Read the model definition and answer for the solid it produces. Units are mm, in the model's axes. A direction names the side the tool comes from. Coordinates: 2 decimals unless noted, no trailing zeros. Write each loop counter-clockwise with the first axis right and the second up, starting at its lowest first coordinate (ties: lowest second). Pieces come first, ordered by that corner, then holes. Notation, with made-up numbers: (76.5, 86.25) -> (130.5, 86.25) arc R29 ccw to (130.5, 120.25) -> close; hole circle Ø11 at (59, -18). An arc over 180 degrees is marked (long way). One line per item, written item: value. Start each with the question number.
1. Find section B-B, the plane x = -111. Write down the section's boundary in (y, z).
2. Find section A-A, the plane x = 106. Write down the section's boundary in (y, z), and give its area (3 significant figures).
3. Consider line 1 along X through (y, z) = (106.5, -475.5); line 2 along X through (y, z) = (-132.5, -267.5); line 3 along X through (y, z) = (83.5, -654). Determine where each line is inside the solid, lowest interval first.
4. For faces 1 (the cylindrical face through (80.64, 126.48, 35.43)), 2 (the flat face through (130, 2, -562)), 3 (the cylindrical face through (142.72, -54.39, -10.21)), 4 (the cylindrical face through (-141.317, -52.335, -9.426)), determine the directions among +Z, -Z, +X, -X, +Y, -Y from which every point of the face is accessible in a straight line to the end or side of a thin tool.
5. For a pull along X with two mould halves and no side action, classify faces 5 (the flat face through (-130, 2, -558)), 6 (the cylindrical face through (140.14, 3.298, -699.964)), 7 (the cylindrical face through (164.297, 143.986, -352.8)) as pulls with the +X half, pulls with the -X half, needs draft (parallel to the pull), parting line crosses it, or undercut.
6. Given P1, Ø1, axis at x = -50.5, y = -93.5, coming from the -Z side; P2, Ø4, axis at x = 72, z = 62.5, coming from the +Y side (3 decimals); P3, Ø3, axis at x = 119, y = 116, coming from the -Z side, each flat-ended and moving along its own axis, determine where each tip first touches the part or whether it passes through.
```python
from build123d import *

# Parameters (mm, degrees)
SKETCH_1_R          = 150
EXTRUDE_1_DEPTH     = 150
EXTRUDE_2_DEPTH     = 170
FILLET_1_R          = 20
FILLET_2_R          = 20
CUT_EXTRUDE_1_DEPTH = 170


with BuildPart() as part:
    # 草图1 → 凸台-拉伸1 (new, symmetric)
    with BuildSketch(Plane.XY):
        Circle(SKETCH_1_R)
    extrude(amount=EXTRUDE_1_DEPTH, both=True)

    # 草图3 → 凸台-拉伸2 (add, symmetric)
    with BuildSketch(Plane(origin=(0, 0, 0), x_dir=(0, 0, -1), z_dir=(1, 0, 0))):
        with BuildLine():
            Line((150, 150), (550, 150))
            ThreePointArc((550, 150), (700, 0), (550, -150))
            Line((550, -150), (150, -150))
            ThreePointArc((150, -150), (0, 0), (150, 150))
        make_face()
    extrude(amount=EXTRUDE_2_DEPTH, both=True)

    # 圆角1
    fillet_1_edges = [part.edges().sort_by_distance(p)[0] for p in [
        (170, -150, -350),
        (170, 150, -350),
        (170, 0, 0),
        (170, 0, -700),
    ]]
    fillet(fillet_1_edges, radius=FILLET_1_R - 0.0001)  # a hair under: the kernel refuses the full size

    # 圆角2
    fillet_2_edges = [part.edges().sort_by_distance(p)[0] for p in [
        (-170, 0, 0),
        (-170, 0, -700),
        (-170, 150, -350),
        (-170, -150, -350),
    ]]
    fillet(fillet_2_edges, radius=FILLET_2_R - 0.0001)  # a hair under: the kernel refuses the full size

    # 草图4 → 切除-拉伸1 (cut, symmetric)
    with BuildSketch(Plane(origin=(0, 0, 0), x_dir=(1, 0, 0), z_dir=(0, 1, 0))):
        with BuildLine():
            Line((-130, 420), (-130, 938.530561272))
            Line((-130, 938.530561272), (130, 938.530561272))
            Line((130, 938.530561272), (130, 420))
            ThreePointArc((130, 420), (0, 290), (-130, 420))
        make_face()
    extrude(amount=CUT_EXTRUDE_1_DEPTH, both=True, mode=Mode.SUBTRACT)


solid = part.part
```
Answer block:
1. outline: (-150, -352.33) -> (150, -352.33) -> (150, -150) arc R150 ccw to (100.89, -39) -> (100.89, 150) -> (-100.89, 150) -> (-100.89, -39) arc R150 ccw to (-150, -150) -> close
2. outline: (-150, -344.74) -> (150, -344.74) -> (150, -150) arc R150 ccw to (106.13, -44) -> (106.13, 150) -> (-106.13, 150) -> (-106.13, -44) arc R150 ccw to (-150, -150) -> close
2. area: 129,000 mm2
3. line 1: x = -170 to -130, 130 to 170
3. line 2: x = -169.84 to 169.84
3. line 3: x = -169.71 to -130, 130 to 169.71
4. face 1: +Z
4. face 2: -Z, +Y, -Y
4. face 3: +Z, +X
4. face 4: +Z, -X
5. face 5: undercut
5. face 6: needs draft
5. face 7: pulls with the +X half
6. P1: stops at z = -300.42
6. P2: stops at y = 132.665
6. P3: stops at z = -371.22
